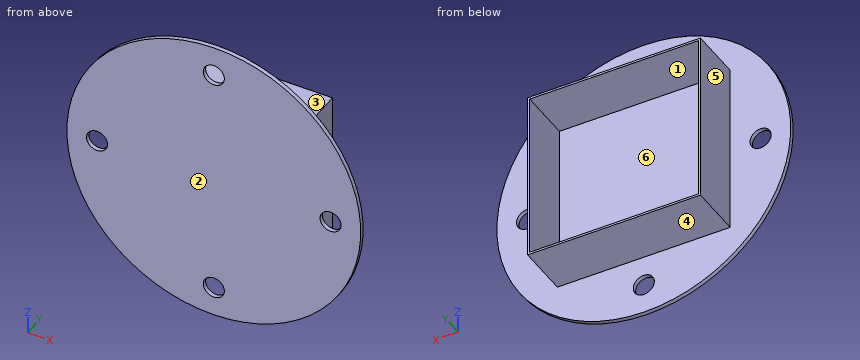
```python
from build123d import *

# Parameters (mm, degrees)
SKETCH1_R           = 88.519
BOSS_EXTRUDE1_DEPTH = 2.54
SKETCH3_W           = 104.14
SKETCH3_H           = 104.14
SKETCH3_W_2         = 101.6
SKETCH3_H_2         = 101.6
BOSS_EXTRUDE2_DEPTH = 31.75
SKETCH4_R           = 6.35
CUT_EXTRUDE1_DEPTH  = 130.148322568


with BuildPart() as part:
    # Sketch1 → Boss-Extrude1 (new body)
    with BuildSketch(Plane(origin=(0, 0, 0), x_dir=(1, 0, 0), z_dir=(0, 1, 0))):
        with Locations(Location((0, 0, 0), (0, 0, 270))):
            Circle(SKETCH1_R)
    extrude(amount=BOSS_EXTRUDE1_DEPTH)

    # Sketch3 → Boss-Extrude2 (add)
    with BuildSketch(Plane(origin=(0, 2.54, 0), x_dir=(1, 0, 0), z_dir=(0, 1, 0))):
        Rectangle(SKETCH3_W, SKETCH3_H)
        Rectangle(SKETCH3_W_2, SKETCH3_H_2, mode=Mode.SUBTRACT)
    extrude(amount=BOSS_EXTRUDE2_DEPTH)

    # Sketch4 → Cut-Extrude1 (cut, through all)
    with BuildSketch(Plane(origin=(0, 2.54, 0), x_dir=(1, 0, 0), z_dir=(0, 1, 0))):
        with Locations(Location((0, 70.4215, 0), (0, 0, 270))):
            Circle(SKETCH4_R)
        with Locations(Location((0, -70.358, 0), (0, 0, 270))):
            Circle(SKETCH4_R)
        with Locations(Location((70.358, 0, 0), (0, 0, 270))):
            Circle(SKETCH4_R)
        with Locations(Location((-70.358, 0, 0), (0, 0, 270))):
            Circle(SKETCH4_R)
    extrude(amount=-CUT_EXTRUDE1_DEPTH, mode=Mode.SUBTRACT)


solid = part.part
```
Model file for the job. Use its own axes, mm. Face numbers are marked on the shaded views. A direction names the side the tool comes from. Give positions to 0.01 mm unless a question says otherwise; leave off trailing zeros. Loops run counter-clockwise (first coordinate to the right, second up) from the corner with the lowest first, then second, coordinate; pieces in that order, holes last. Notation, with made-up numbers: (84.5, -35.75) -> (111.5, -35.75) arc R13 ccw to (111.5, -21.75) -> close; hole circle Ø3 at (89, 19.5). An arc over 180 degrees is marked (long way). Write each question's results on one line, items separated by ' | '.
(1) Cut at B-B on x = 0. List the corners of the cut face in (y, z).
Geometry results:
outline: (0, -88.52) -> (2.54, -88.52) -> (2.54, -76.77) -> (0, -76.77) -> close; (0, -64.07) -> (2.54, -64.07) -> (2.54, -52.07) -> (34.29, -52.07) -> (34.29, -50.8) -> (2.54, -50.8) -> (2.54, 50.8) -> (34.29, 50.8) -> (34.29, 52.07) -> (2.54, 52.07) -> (2.54, 64.01) -> (0, 64.01) -> close; (0, 76.71) -> (2.54, 76.71) -> (2.54, 88.52) -> (0, 88.52) -> close
(2) Probe line 1 along X through (y, z) = (12.5, -49.5); line 2 along X through (y, z) = (1.5, 0). List the from-to ranges inside material, lowest first.
Geometry results:
line 1: x = -52.07 to -50.8, 50.8 to 52.07 | line 2: x = -88.52 to -76.71, -64.01 to 64.01, 76.71 to 88.52
(3) Pull direction X, two halves, no side cores. Call the marked faces 4, 5 and 6: released by +X, released by -X, zero draft, split by the parting line, or undercut.
Geometry results:
face 4: zero draft | face 5: released by -X | face 6: undercut
(4) Cut at C-C on y = 25.5. List the corners of the cut face in (x, z).
Geometry results:
outline: (-52.07, -52.07) -> (52.07, -52.07) -> (52.07, 52.07) -> (-52.07, 52.07) -> close; hole (-50.8, -50.8) -> (50.8, -50.8) -> (50.8, 50.8) -> (-50.8, 50.8) -> close
(5) Tool access for the marked faces 1, 2 and 3: list every direction of +Z, -Z, +X, -X, +Y, -Y with a clear straight run to the whole face (end or side of a thin tool).
Geometry results:
face 1: +Y | face 2: +Z, -Z, +X, -X, -Y | face 3: +Z, +X, -X, +Y
(6) Flat gauge pins, fed straight in: pin 1 Ø1 at (x, y) = (-16, 11.5) entering from -Z; pin 2 Ø9.5 at (y, z) = (22, 4.5) entering from -X; pin 3 Ø20.5 at (x, z) = (-70.358, 0) entering from +Y. Where does each tip first touch, or does it go through?
Geometry results:
pin 1: stops at z = -52.07 | pin 2: stops at x = -52.07 | pin 3: stops at y = 2.54
(7) Cut at A-A on z = 0. List the corners of the cut face in (x, y).
Geometry results:
outline: (-88.52, 0) -> (-76.71, 0) -> (-76.71, 2.54) -> (-88.52, 2.54) -> close; (-64.01, 0) -> (64.01, 0) -> (64.01, 2.54) -> (52.07, 2.54) -> (52.07, 34.29) -> (50.8, 34.29) -> (50.8, 2.54) -> (-50.8, 2.54) -> (-50.8, 34.29) -> (-52.07, 34.29) -> (-52.07, 2.54) -> (-64.01, 2.54) -> close; (76.71, 0) -> (88.52, 0) -> (88.52, 2.54) -> (76.71, 2.54) -> close
(8) Cut at D-D on z = 26.5. List the corners of the cut face in (x, y).
Geometry results:
outline: (-84.46, 0) -> (84.46, 0) -> (84.46, 2.54) -> (52.07, 2.54) -> (52.07, 34.29) -> (50.8, 34.29) -> (50.8, 2.54) -> (-50.8, 2.54) -> (-50.8, 34.29) -> (-52.07, 34.29) -> (-52.07, 2.54) -> (-84.46, 2.54) -> close
